Part model, mm, in its own coordinate system. A direction names the side the tool comes from. Give positions to 0.01 mm unless a question says otherwise; leave off trailing zeros. Write each loop counter-clockwise with the first axis right and the second up, starting at its lowest first coordinate (ties: lowest second). Pieces come first, ordered by that corner, then holes. Notation, with made-up numbers: M 37,12.25 L 81,12.25 A33 ccw 81,45.25 Z; hole C 1.25,12 d3. An arc over 180 degrees is marked long. Use a Markdown table: item, result.
```python
from build123d import *

# Parameters (mm, degrees)
F0_W     = 35
F0_H     = 32
F1_DEPTH = 11
F2_W     = 35
F2_H     = 28.5
F3_DEPTH = 4
F4_R     = 1.25
F5_DEPTH = 25
F6_R     = 2.15
F7_DEPTH = 3


with BuildPart() as f1:
    # F0 (on Top) → F1 (new body)
    with BuildSketch(Plane.XY):
        with Locations((17.5, 16)):
            Rectangle(F0_W, F0_H)
    extrude(amount=F1_DEPTH)

    # F2 (on face) → F3 (cut)
    with BuildSketch(Plane.XY.offset(11)):
        with Locations((17.5, 16)):
            Rectangle(F2_W, F2_H)
    extrude(amount=-F3_DEPTH, mode=Mode.SUBTRACT)

    # F4 (on face) → F5 (cut)
    with BuildSketch(Plane.XY.offset(7)):
        with Locations((6, 22)):
            Circle(F4_R)
        with Locations((6, 10)):
            Circle(F4_R)
        with Locations((14, 22)):
            Circle(F4_R)
        with Locations((14, 10)):
            Circle(F4_R)
        with Locations((16, 27)):
            Circle(F4_R)
        with Locations((16, 5)):
            Circle(F4_R)
    extrude(amount=-F5_DEPTH, mode=Mode.SUBTRACT)

    # F6 (on face) → F7 (cut)
    with BuildSketch(Plane.XY.offset(7)):
        with Locations((6, 22)):
            Circle(F6_R)
        with Locations((14, 22)):
            Circle(F6_R)
        with Locations((14, 10)):
            Circle(F6_R)
        with Locations((6, 10)):
            Circle(F6_R)
    extrude(amount=-F7_DEPTH, mode=Mode.SUBTRACT)


solid = f1.part
```
1. Cut at C-C, the plane z = 2.5. Give the cut face in (x, y).
Findings below:
| item | result |
|---|---|
| outline | M 0,0 L 35,0 L 35,32 L 0,32 Z; hole C 6,10 d2.5; hole C 6,22 d2.5; hole C 14,10 d2.5; hole C 14,22 d2.5; hole C 16,5 d2.5; hole C 16,27 d2.5 |
2. Drill centre lines: L1, parallel to Y at x = 14, z = 6.2; L2, parallel to Y at x = 6, z = 1.9; L3, parallel to Y at x = 18.5, z = 9. Where is each one in solid material? Low to high.
Findings below:
| item | result |
|---|---|
| L1 | 0 to 7.85, 12.15 to 19.85, 24.15 to 32 |
| L2 | 0 to 8.75, 11.25 to 20.75, 23.25 to 32 |
| L3 | 0 to 1.75, 30.25 to 32 |
3. Drop flat-ended pins along their axis: P1, Ø6, axis at x = 25.5, y = 8, coming from the +Z side; P2, Ø2, axis at x = 6, y = 10, coming from the +Z side; P3, Ø1.3, axis at x = 13.5, y = 9, coming from the +Z side. Give the stop position or say it passes through.
Findings below:
| item | result |
|---|---|
| P1 | z = 7 |
| P2 | through |
| P3 | z = 4 |
4. Cut at D-D, the plane y = 22. Give the cut face in (x, z).
Findings below:
| item | result |
|---|---|
| outline | M 0,0 L 4.75,0 L 4.75,4 L 3.85,4 L 3.85,7 L 0,7 Z; M 7.25,0 L 12.75,0 L 12.75,4 L 11.85,4 L 11.85,7 L 8.15,7 L 8.15,4 L 7.25,4 Z; M 15.25,0 L 35,0 L 35,7 L 16.15,7 L 16.15,4 L 15.25,4 Z |
5. Cut at A-A, the plane y = 5. Give the cut face in (x, z), then the cut area to 4 significant figures.
Findings below:
| item | result |
|---|---|
| outline | M 0,0 L 14.75,0 L 14.75,7 L 0,7 Z; M 17.25,0 L 35,0 L 35,7 L 17.25,7 Z |
| area | 227.5 mm2 |
6. Two-plate mould, pull along Y, no slides. Class faces 4 (the flat face through (17, 32, 5)), 5 (the flat face through (17, 31, 11)), 6 (the flat face through (7, 21, 4)): released by +Y, released by -Y, zero draft, split by the parting line, or undercut.
Findings below:
| item | result |
|---|---|
| face 4 | released by +Y |
| face 5 | zero draft |
| face 6 | undercut |
7. Tool access for faces 1 (the flat face through (17, 30.25, 9)), 2 (the cylindrical face through (15.73, 3.78, 3.55)), 3 (the cylindrical face through (4.294, 20.692, 5.521)): list every direction of +Z, -Z, +X, -X, +Y, -Y with a clear straight run to the whole face (end or side of a thin tool).
Findings below:
| item | result |
|---|---|
| face 1 | +Z, +X, -X |
| face 2 | +Z, -Z |
| face 3 | +Z |
8. Cut at B-B, the plane x = 6. Give the cut face in (y, z).
Findings below:
| item | result |
|---|---|
| outline | M 0,0 L 8.75,0 L 8.75,4 L 7.85,4 L 7.85,7 L 1.75,7 L 1.75,11 L 0,11 Z; M 11.25,0 L 20.75,0 L 20.75,4 L 19.85,4 L 19.85,7 L 12.15,7 L 12.15,4 L 11.25,4 Z; M 23.25,0 L 32,0 L 32,11 L 30.25,11 L 30.25,7 L 24.15,7 L 24.15,4 L 23.25,4 Z |
